Geometry check sheet. Reference: the model listing, model coordinates, mm. Face numbers are marked on the shaded views. A direction names the side the tool comes from. Give positions to 0.01 mm unless a question says otherwise; leave off trailing zeros. Write each loop counter-clockwise with the first axis right and the second up, starting at its lowest first coordinate (ties: lowest second). Pieces come first, ordered by that corner, then holes. Notation, with made-up numbers: (-38, 39) -> (-23, 39) arc R20 cw to (-23, 45) -> close; hole circle Ø9 at (-3.5, -7.5). An arc over 180 degrees is marked (long way). One line per item, written item: value.
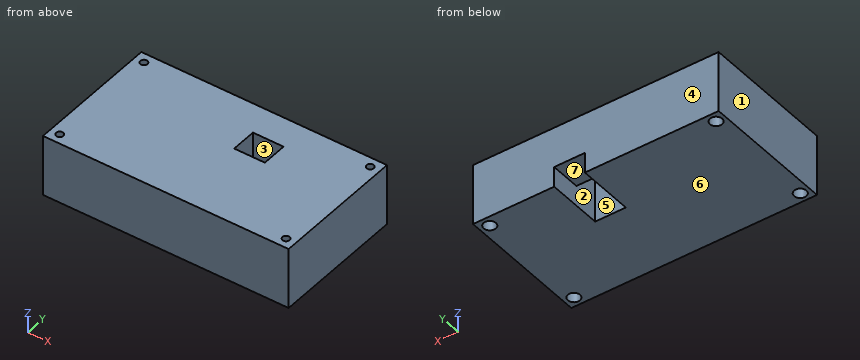
from build123d import *

# Parameters (mm, degrees)
SKETCH008_W         = 120.815
SKETCH008_H         = 65.873
PAD004_DEPTH        = 30
HOLE002_D           = 3.5
HOLE002_CBORE_D     = 6
HOLE002_CBORE_DEPTH = 20
SKETCH010_W         = 15.08
SKETCH010_H         = 12.54
POCKET002_DEPTH     = 30.001
SKETCH011_W         = 15.08
SKETCH011_H         = 14.883
POCKET003_DEPTH     = 10


with BuildPart() as part:
    # Sketch008 (on Face1 of Binder002) → Pad004 (new body)
    with BuildSketch(Plane(origin=(0, 0, -35), x_dir=(1, 0, 0), z_dir=(0, 0, -1))):
        with Locations((50.4075, -22.9365)):
            Rectangle(SKETCH008_W, SKETCH008_H)
    extrude(amount=PAD004_DEPTH)

    # Hole002 (through all)
    with Locations(Plane(origin=(0, 0, -65), x_dir=(1, 0, 0), z_dir=(0, 0, -1))):
        with Locations((-5.25, 5.25), (106.065, 5.25), (106.065, -51.123), (-5.25, -51.123)):
            CounterBoreHole(HOLE002_D / 2, HOLE002_CBORE_D / 2, HOLE002_CBORE_DEPTH)

    # Sketch010 (on Face5 of Hole002) → Pocket002 (cut, through all)
    with BuildSketch(Plane(origin=(0, 0, -65), x_dir=(1, 0, 0), z_dir=(0, 0, -1))):
        with Locations((63.34, -34.72)):
            Rectangle(SKETCH010_W, SKETCH010_H)
    extrude(amount=-POCKET002_DEPTH, mode=Mode.SUBTRACT)

    # Sketch011 (on Face5 of Pocket002) → Pocket003 (cut)
    with BuildSketch(Plane(origin=(0, 0, -65), x_dir=(1, 0, 0), z_dir=(0, 0, -1))):
        with Locations((63.34, -48.4315)):
            Rectangle(SKETCH011_W, SKETCH011_H)
    extrude(amount=-POCKET003_DEPTH, mode=Mode.SUBTRACT)


solid = part.part
1) Sectioned sample at C-C on z = -41. Record the cut outline in (x, y) (3 decimals), plus the area to 3 significant figures.
Verdict:
outline: (-10, -10) -> (110.815, -10) -> (110.815, 55.873) -> (-10, 55.873) -> close; hole circle Ø3.5 at (-5.25, -5.25); hole circle Ø3.5 at (-5.25, 51.123); hole (55.8, 28.45) -> (70.88, 28.45) -> (70.88, 40.99) -> (55.8, 40.99) -> close; hole circle Ø3.5 at (106.065, -5.25); hole circle Ø3.5 at (106.065, 51.123)
area: 7,730 mm^2
2) Scan lines: probe 1 along Y at (x, z) = (-5.25, -53); probe 2 along Y at (x, z) = (-5.25, -42); probe 3 along X at (y, z) = (32, -38.25) (3 decimals). Record each from-to range of solid material in increasing order.
Verdict:
probe 1: -10 to -8.25, -2.25 to 48.12, 54.12 to 55.87
probe 2: -10 to -7, -3.5 to 49.37, 52.87 to 55.87
probe 3: -10 to 55.8, 70.88 to 110.815
3) Sectioned sample at A-A on x = -5.25. Record the cut outline in (y, z), plus the area to 3 significant figures.
Verdict:
outline: (-10, -65) -> (-8.25, -65) -> (-8.25, -45) -> (-7, -45) -> (-7, -35) -> (-10, -35) -> close; (-3.5, -45) -> (-2.25, -45) -> (-2.25, -65) -> (48.12, -65) -> (48.12, -45) -> (49.37, -45) -> (49.37, -35) -> (-3.5, -35) -> close; (52.87, -45) -> (54.12, -45) -> (54.12, -65) -> (55.87, -65) -> (55.87, -35) -> (52.87, -35) -> close
area: 1,670 mm^2
4) Mould release check, pull along Y, two halves, no side actions. Record for the marked faces 1, 2, 3 and 4: released by +Y, released by -Y, zero draft, split by the parting line, or undercut.
Verdict:
face 1: zero draft
face 2: undercut
face 3: undercut
face 4: released by +Y
5) Depth check by flat-ended pin: pin 1 Ø5 at (x, y) = (-5.25, 51.123) entering from -Z; pin 2 Ø2 at (x, y) = (106.065, -5.25) entering from -Z. Enter the tip coordinate at first touch or a pass-through.
Verdict:
pin 1: z = -45
pin 2: through
6) Tool access check on the marked faces 5, 6 and 7. Record the directions out of +Z, -Z, +X, -X, +Y, -Y that give a thin tool (end or side, any length) a straight path to the whole face; none if there is none.
Verdict:
face 5: +Z, -Z
face 6: -Z, +X, -X, +Y, -Y
face 7: -Z, +Y
7) Sectioned sample at B-B on y = -5.25. Record the cut outline in (x, z) (3 decimals), plus the area to 3 significant figures.
Verdict:
outline: (-10, -65) -> (-8.25, -65) -> (-8.25, -45) -> (-7, -45) -> (-7, -35) -> (-10, -35) -> close; (-3.5, -45) -> (-2.25, -45) -> (-2.25, -65) -> (103.065, -65) -> (103.065, -45) -> (104.315, -45) -> (104.315, -35) -> (-3.5, -35) -> close; (107.815, -45) -> (109.065, -45) -> (109.065, -65) -> (110.815, -65) -> (110.815, -35) -> (107.815, -35) -> close
area: 3,310 mm^2
